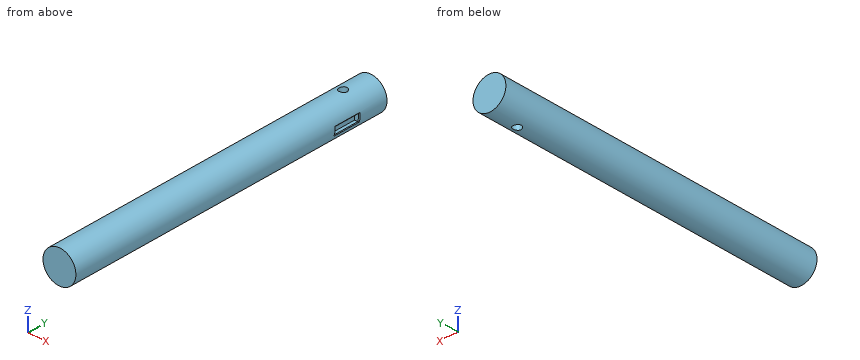
```python
from build123d import *

# Parameters (mm, degrees)
CROQUIS1_R                 = 19.05
SALIENTE_EXTRUIR1_DEPTH    = 394
CORTAR_EXTRUIR1_DEPTH      = 395.919998227
CORTAR_EXTRUIR1_DEPTH_BACK = 395.919998227
CROQUIS2_R                 = 4.765
CORTAR_EXTRUIR2_DEPTH      = 397.295991136
CORTAR_EXTRUIR2_DEPTH_BACK = 5.45
CROQUIS4_W                 = 8.29
CROQUIS4_H                 = 29.8
CHAFL_N1_SIZE              = 1
CHAFL_N1_SIZE_2            = 0.898769363
CHAFL_N1_SIZE_3            = 0.790943361


with BuildPart() as part:
    # Croquis1 → Saliente-Extruir1 (new body)
    with BuildSketch(Plane(origin=(0, 0, 0), x_dir=(1, 0, 0), z_dir=(0, 1, 0))):
        with Locations(Location((0, 0, 0), (0, 0, 270))):
            Circle(CROQUIS1_R)
    extrude(amount=SALIENTE_EXTRUIR1_DEPTH)

    # Croquis2 → Cortar-Extruir1 (cut, two sides: drawn at the far end of the back side and taken through both)
    with BuildSketch(Plane.XY.offset(-CORTAR_EXTRUIR1_DEPTH_BACK)):
        with Locations(Location((0, 359, 0), (0, 0, 90.000000003))):
            Circle(CROQUIS2_R)
    extrude(amount=CORTAR_EXTRUIR1_DEPTH + CORTAR_EXTRUIR1_DEPTH_BACK, mode=Mode.SUBTRACT)

    # Croquis4 → Cortar-Extruir2 (cut, two sides: drawn at the far end of the back side and taken through both)
    with BuildSketch(Plane(origin=(19.05, 0, 0), x_dir=(0, 0, -1), z_dir=(1, 0, 0)).offset(-CORTAR_EXTRUIR2_DEPTH_BACK)):
        with Locations((1.862063648, 344.1)):
            Rectangle(CROQUIS4_W, CROQUIS4_H)
    extrude(amount=CORTAR_EXTRUIR2_DEPTH + CORTAR_EXTRUIR2_DEPTH_BACK, mode=Mode.SUBTRACT)

    # Chaflán1
    # the kernel refuses this chamfer: 1, 0.898769363, 0.790943361 mm, written as the material it takes off along each edge
    with BuildSketch(Plane(origin=(0, 329.2, 0), x_dir=(0.8979062520865971, 0, -0.4401867359017083), z_dir=(-0.4401867359017083, 0, -0.8979062520865971))) as chafl_n1_piece_1_section:
        Polygon((19.05, CHAFL_N1_SIZE), (19.05 - CHAFL_N1_SIZE, 0), (19.05, 0), align=None)
    chafl_n1_piece_1 = revolve(axis=Axis((0, 329.2, 0), (0, -1, 0)), revolution_arc=40.733590892, mode=Mode.PRIVATE)
    chafl_n1_piece_1 = split(chafl_n1_piece_1, bisect_by=Plane(origin=(0, 329.2, 2.282936352), z_dir=(0, 0, -1)), keep=Keep.TOP, mode=Mode.PRIVATE)
    chafl_n1_piece_1 = split(chafl_n1_piece_1, bisect_by=Plane(origin=(0, 329.2, -6.007063648), z_dir=(0, 0, 1)), keep=Keep.TOP, mode=Mode.PRIVATE)
    add(chafl_n1_piece_1, mode=Mode.SUBTRACT)
    with BuildSketch(Plane(origin=(0, 359, 0), x_dir=(0.8979062520865971, 0, -0.4401867359017083), z_dir=(-0.4401867359017083, 0, -0.8979062520865971))) as chafl_n1_piece_2_section:
        Polygon((19.05, -CHAFL_N1_SIZE), (19.05 - CHAFL_N1_SIZE, 0), (19.05, 0), align=None)
    chafl_n1_piece_2 = revolve(axis=Axis((0, 359, 0), (0, -1, 0)), revolution_arc=40.733590892, mode=Mode.PRIVATE)
    chafl_n1_piece_2 = split(chafl_n1_piece_2, bisect_by=Plane(origin=(0, 359, 2.282936352), z_dir=(0, 0, -1)), keep=Keep.TOP, mode=Mode.PRIVATE)
    chafl_n1_piece_2 = split(chafl_n1_piece_2, bisect_by=Plane(origin=(0, 359, -6.007063648), z_dir=(0, 0, 1)), keep=Keep.TOP, mode=Mode.PRIVATE)
    add(chafl_n1_piece_2, mode=Mode.SUBTRACT)
    with BuildSketch(Plane(origin=(18.912712698, 359, 2.282936352), x_dir=(-0.1452151757871569, 0, 0.9894000973929127), z_dir=(0, -1, 0))) as chafl_n1_piece_3:
        with BuildLine():
            Line((0.975350899, 0), (CHAFL_N1_SIZE_2 * 0.14521517582, CHAFL_N1_SIZE_2 * 0.989400097614))
            Line((CHAFL_N1_SIZE_2 * 0.14521517582, CHAFL_N1_SIZE_2 * 0.989400097614), (0, 0))
            ThreePointArc((0, 0), (0.501444944, -0.006238234), (0.975350899, 0))
        make_face()
    extrude(amount=29.8, mode=Mode.SUBTRACT)
    with BuildSketch(Plane(origin=(18.078099633, 359, -6.007063648), x_dir=(-0.33952178475198846, 0, -0.9405981914073748), z_dir=(0, -1, 0))) as chafl_n1_piece_4:
        with BuildLine():
            Line((0.975350899, 0), (CHAFL_N1_SIZE_3 * 0.339521784837, -CHAFL_N1_SIZE_3 * 0.940598191643))
            Line((CHAFL_N1_SIZE_3 * 0.339521784837, -CHAFL_N1_SIZE_3 * 0.940598191643), (0, 0))
            ThreePointArc((0, 0), (0.501444944, 0.006238234), (0.975350899, 0))
        make_face()
    extrude(amount=29.8, mode=Mode.SUBTRACT)
    with BuildSketch(Plane(origin=(0, 329.2, 0), x_dir=(0.8979062520865971, 0, -0.4401867359017083), z_dir=(-0.4401867359017083, 0, -0.8979062520865971))) as chafl_n1_piece_5a_section:
        Polygon((19.05, CHAFL_N1_SIZE), (19.05 - CHAFL_N1_SIZE, 0), (19.05, 0), align=None)
    chafl_n1_piece_5a = revolve(axis=Axis((0, 329.2, 0), (0, -1, 0)), revolution_arc=40.733590892, mode=Mode.PRIVATE)
    chafl_n1_piece_5a = split(chafl_n1_piece_5a, bisect_by=Plane(origin=(0, 329.2, -6.007063648), z_dir=(0, 0, -1)), keep=Keep.TOP, mode=Mode.PRIVATE)
    with BuildSketch(Plane(origin=(18.078099633, 359, -6.007063648), x_dir=(-0.33952178475198846, 0, -0.9405981914073748), z_dir=(0, -1, 0))) as chafl_n1_piece_5b_section:
        with BuildLine():
            Line((0.975350899, 0), (CHAFL_N1_SIZE_3 * 0.339521784837, -CHAFL_N1_SIZE_3 * 0.940598191643))
            Line((CHAFL_N1_SIZE_3 * 0.339521784837, -CHAFL_N1_SIZE_3 * 0.940598191643), (0, 0))
            ThreePointArc((0, 0), (0.501444944, 0.006238234), (0.975350899, 0))
        make_face()
    chafl_n1_piece_5b = extrude(amount=32.308302498, mode=Mode.PRIVATE)
    chafl_n1_piece_5b = split(chafl_n1_piece_5b, bisect_by=Plane(origin=(18.078099633, 329.2, -6.007063648), z_dir=(0, -1, 0)), keep=Keep.TOP, mode=Mode.PRIVATE)
    chafl_n1_piece_5 = chafl_n1_piece_5a & chafl_n1_piece_5b
    add(chafl_n1_piece_5, mode=Mode.SUBTRACT)
    with BuildSketch(Plane(origin=(0, 329.2, 0), x_dir=(0.8979062520865971, 0, -0.4401867359017083), z_dir=(-0.4401867359017083, 0, -0.8979062520865971))) as chafl_n1_piece_6a_section:
        Polygon((19.05, CHAFL_N1_SIZE), (19.05 - CHAFL_N1_SIZE, 0), (19.05, 0), align=None)
    chafl_n1_piece_6a = revolve(axis=Axis((0, 329.2, 0), (0, -1, 0)), revolution_arc=40.733590892, mode=Mode.PRIVATE)
    chafl_n1_piece_6a = split(chafl_n1_piece_6a, bisect_by=Plane(origin=(0, 329.2, 2.282936352), z_dir=(0, 0, 1)), keep=Keep.TOP, mode=Mode.PRIVATE)
    with BuildSketch(Plane(origin=(18.912712698, 359, 2.282936352), x_dir=(-0.1452151757871569, 0, 0.9894000973929127), z_dir=(0, -1, 0))) as chafl_n1_piece_6b_section:
        with BuildLine():
            Line((0.975350899, 0), (CHAFL_N1_SIZE_2 * 0.14521517582, CHAFL_N1_SIZE_2 * 0.989400097614))
            Line((CHAFL_N1_SIZE_2 * 0.14521517582, CHAFL_N1_SIZE_2 * 0.989400097614), (0, 0))
            ThreePointArc((0, 0), (0.501444944, -0.006238234), (0.975350899, 0))
        make_face()
    chafl_n1_piece_6b = extrude(amount=32.308302498, mode=Mode.PRIVATE)
    chafl_n1_piece_6b = split(chafl_n1_piece_6b, bisect_by=Plane(origin=(18.912712698, 329.2, 2.282936352), z_dir=(0, -1, 0)), keep=Keep.TOP, mode=Mode.PRIVATE)
    chafl_n1_piece_6 = chafl_n1_piece_6a & chafl_n1_piece_6b
    add(chafl_n1_piece_6, mode=Mode.SUBTRACT)
    with BuildSketch(Plane(origin=(0, 359, 0), x_dir=(0.8979062520865971, 0, -0.4401867359017083), z_dir=(-0.4401867359017083, 0, -0.8979062520865971))) as chafl_n1_piece_7a_section:
        Polygon((19.05, -CHAFL_N1_SIZE), (19.05 - CHAFL_N1_SIZE, 0), (19.05, 0), align=None)
    chafl_n1_piece_7a = revolve(axis=Axis((0, 359, 0), (0, -1, 0)), revolution_arc=40.733590892, mode=Mode.PRIVATE)
    chafl_n1_piece_7a = split(chafl_n1_piece_7a, bisect_by=Plane(origin=(0, 359, -6.007063648), z_dir=(0, 0, -1)), keep=Keep.TOP, mode=Mode.PRIVATE)
    with BuildSketch(Plane(origin=(18.078099633, 361.508302498, -6.007063648), x_dir=(-0.33952178475198846, 0, -0.9405981914073748), z_dir=(0, -1, 0))) as chafl_n1_piece_7b_section:
        with BuildLine():
            Line((0.975350899, 0), (CHAFL_N1_SIZE_3 * 0.339521784837, -CHAFL_N1_SIZE_3 * 0.940598191643))
            Line((CHAFL_N1_SIZE_3 * 0.339521784837, -CHAFL_N1_SIZE_3 * 0.940598191643), (0, 0))
            ThreePointArc((0, 0), (0.501444944, 0.006238234), (0.975350899, 0))
        make_face()
    chafl_n1_piece_7b = extrude(amount=32.308302498, mode=Mode.PRIVATE)
    chafl_n1_piece_7b = split(chafl_n1_piece_7b, bisect_by=Plane(origin=(18.078099633, 359, -6.007063648), z_dir=(0, 1, 0)), keep=Keep.TOP, mode=Mode.PRIVATE)
    chafl_n1_piece_7 = chafl_n1_piece_7a & chafl_n1_piece_7b
    add(chafl_n1_piece_7, mode=Mode.SUBTRACT)
    with BuildSketch(Plane(origin=(18.912712698, 361.508302498, 2.282936352), x_dir=(-0.1452151757871569, 0, 0.9894000973929127), z_dir=(0, -1, 0))) as chafl_n1_piece_8a_section:
        with BuildLine():
            Line((0.975350899, 0), (CHAFL_N1_SIZE_2 * 0.14521517582, CHAFL_N1_SIZE_2 * 0.989400097614))
            Line((CHAFL_N1_SIZE_2 * 0.14521517582, CHAFL_N1_SIZE_2 * 0.989400097614), (0, 0))
            ThreePointArc((0, 0), (0.501444944, -0.006238234), (0.975350899, 0))
        make_face()
    chafl_n1_piece_8a = extrude(amount=32.308302498, mode=Mode.PRIVATE)
    chafl_n1_piece_8a = split(chafl_n1_piece_8a, bisect_by=Plane(origin=(18.912712698, 359, 2.282936352), z_dir=(0, 1, 0)), keep=Keep.TOP, mode=Mode.PRIVATE)
    with BuildSketch(Plane(origin=(0, 359, 0), x_dir=(0.8979062520865971, 0, -0.4401867359017083), z_dir=(-0.4401867359017083, 0, -0.8979062520865971))) as chafl_n1_piece_8b_section:
        Polygon((19.05, -CHAFL_N1_SIZE), (19.05 - CHAFL_N1_SIZE, 0), (19.05, 0), align=None)
    chafl_n1_piece_8b = revolve(axis=Axis((0, 359, 0), (0, -1, 0)), revolution_arc=40.733590892, mode=Mode.PRIVATE)
    chafl_n1_piece_8b = split(chafl_n1_piece_8b, bisect_by=Plane(origin=(0, 359, 2.282936352), z_dir=(0, 0, 1)), keep=Keep.TOP, mode=Mode.PRIVATE)
    chafl_n1_piece_8 = chafl_n1_piece_8a & chafl_n1_piece_8b
    add(chafl_n1_piece_8, mode=Mode.SUBTRACT)


solid = part.part
```
Verification items for the finished model (mm, model axes). Coordinates: 2 decimals unless noted, no trailing zeros. Order: outer loops, then holes, each group sorted by start corner. A loop starts at its lowest first (then second) coordinate and runs counter-clockwise, first axis right, second up. Notation, with made-up numbers: (84.5, -15.75) -> (137.5, -15.75) arc R31 cw to (137.5, 20.25) -> close; hole circle Ø3 at (33, 34.25). An arc over 180 degrees is marked (long way). Put each result on its own line as item: value. Start each with the question number.
1) Material ranges on L1, parallel to Y at x = 0, z = -2 (3 decimals); L2, parallel to X at y = 359, z = -8 (3 decimals); L3, parallel to X at y = 359, z = 9 (3 decimals), recorded low to high.
2) Cross-section at B-B (z = 14.5). Enter the section's corners in (x, y) (3 decimals).
3) Go/stop test with flat-tipped pins: pin 1 (1.5 mm diameter, centred on x = 14.5, y = 124.5, fed in from +Z); pin 2 (4 mm diameter, centred on x = 15, y = 342, fed in from +Z); pin 3 (6 mm diameter, centred on y = 332.5, z = 3.5, fed in from +X); pin 4 (5.5 mm diameter, centred on x = 0, y = 359, fed in from -Z). Record where each tip stops, or that it passes through.
4) Cross-section at A-A (x = 0). Enter the section's corners in (y, z) (3 decimals), plus the area to 3 significant figures.
5) Cross-section at D-D (x = -14.5). Enter the section's corners in (y, z).
6) Cross-section at C-C (y = 336.5). Enter the section's corners in (x, z).
Geometry check:
1. L1: y = 0 to 354.235, 363.765 to 394
1. L2: x = -17.289 to -4.765, 4.765 to 17.289
1. L3: x = -16.79 to -4.765, 4.765 to 16.79
2. outline: (-12.355, 0) -> (12.355, 0) -> (12.355, 394) -> (-12.355, 394) -> close; hole circle Ø9.53 at (0, 359)
3. pin 1: stops at z = 13.18
3. pin 2: stops at z = 13.92
3. pin 3: stops at x = 18.77
3. pin 4: passes through
4. outline: (0, -19.05) -> (354.235, -19.05) -> (354.235, 19.05) -> (0, 19.05) -> close; (363.765, -19.05) -> (394, -19.05) -> (394, 19.05) -> (363.765, 19.05) -> close
4. area: 14,600 mm^2
5. outline: (0, -12.36) -> (394, -12.36) -> (394, 12.36) -> (0, 12.36) -> close
6. outline: (13.6, -6.01) -> (13.6, 2.28) -> (18.01, 2.28) -> (18.77, 3.25) arc R19.05 ccw (long way) to (17.75, -6.92) -> (17.29, -6.01) -> close
